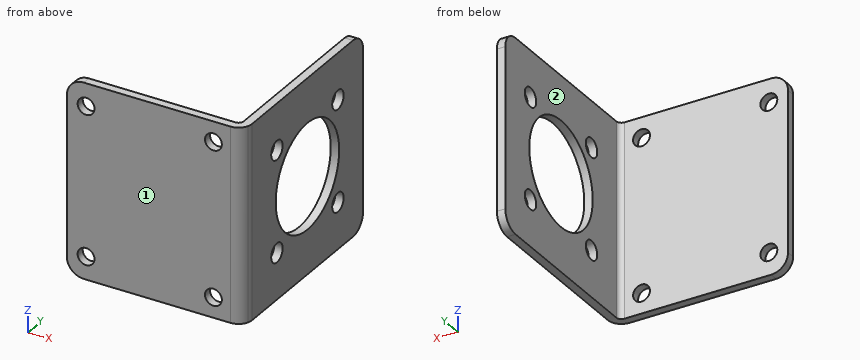
from build123d import *

# Parameters (mm, degrees)
BASE_FLANGE1_DEPTH     = 2
SKETCHED_START         = -23
SKETCHED_BEND1_DEPTH   = 46
SKETCHED_BEND1_2_DEPTH = 46
SKETCH7_R              = 12.5
SKETCH7_R_2            = 2.25
CUT_EXTRUDE1_DEPTH     = 2
SKETCH8_R              = 2
CUT_EXTRUDE2_DEPTH     = 2
FILLET1_R              = 4


# Read off the part's stored shape, not the designer's step: Sketched Bend1
# Sheet-metal steps are written as plain solids
with BuildPart() as part:
    # Sketch1 → Base-Flange1 (new body)
    with BuildSketch(Plane(origin=(0, 0, 0), x_dir=(1, 0, 0), z_dir=(0, 1, 0))):
        Polygon((-20, 23), (20, 23), (66, 23), (66, -23), (20, -23), (-20, -23), align=None)
    extrude(amount=-BASE_FLANGE1_DEPTH)

    # Sketched Bend1 outline → Sketched Bend1 (cut)
    with BuildSketch(Plane.XY.offset(SKETCHED_START)):
        with BuildLine():
            Line((66, 0), (21.766479395, 0))
            ThreePointArc((21.766479395, 0), (20.588854382, -1.453299832), (18.8, -2))
            Line((18.8, -2), (66, -2))
            Line((66, -2), (66, 0))
        make_face()
    extrude(amount=SKETCHED_BEND1_DEPTH, mode=Mode.SUBTRACT)

    # Sketched Bend1 2 outline → Sketched Bend1 2 (add)
    with BuildSketch(Plane.XY.offset(SKETCHED_START)):
        with BuildLine():
            Line((20, 44.944248081), (20, 1.2))
            ThreePointArc((20, 1.2), (19.648528137, 0.351471863), (18.8, 0))
            Line((18.8, 0), (21.766479395, 0))
            ThreePointArc((21.766479395, 0), (21.941077368, 0.58874476), (22, 1.2))
            Line((22, 1.2), (22, 44.944248081))
            Line((22, 44.944248081), (20, 44.944248081))
        make_face()
    extrude(amount=SKETCHED_BEND1_2_DEPTH)

    # Sketch7 → Cut-Extrude1 (cut)
    with BuildSketch(Plane(origin=(22, 0, 0), x_dir=(0, 0, -1), z_dir=(1, 0, 0))):
        with Locations(Location((0, 23, 0), (0, 0, 90))):
            Circle(SKETCH7_R)
        with Locations(Location((12.02081528, 35.02081528, 0), (0, 0, 90))):
            Circle(SKETCH7_R_2)
        with Locations(Location((12.02081528, 10.97918472, 0), (0, 0, 90))):
            Circle(SKETCH7_R_2)
        with Locations(Location((-12.02081528, 10.97918472, 0), (0, 0, 90))):
            Circle(SKETCH7_R_2)
        with Locations(Location((-12.02081528, 35.02081528, 0), (0, 0, 90))):
            Circle(SKETCH7_R_2)
    extrude(amount=-CUT_EXTRUDE1_DEPTH, mode=Mode.SUBTRACT)

    # Sketch8 → Cut-Extrude2 (cut)
    with BuildSketch(Plane(origin=(0, 0, 0), x_dir=(1, 0, 0), z_dir=(0, 1, 0))):
        with Locations(Location((-15.450942979, 17.606788068, 0), (0, 0, 270))):
            Circle(SKETCH8_R)
        with Locations(Location((-15.450942979, -17.606788068, 0), (0, 0, 90))):
            Circle(SKETCH8_R)
        with Locations(Location((14.749785428, 18.198199219, 0), (0, 0, 270))):
            Circle(SKETCH8_R)
        with Locations(Location((14.749785428, -18.198199219, 0), (0, 0, 90))):
            Circle(SKETCH8_R)
    extrude(amount=-CUT_EXTRUDE2_DEPTH, mode=Mode.SUBTRACT)

    # Fillet1
    fillet1_edges = [part.edges().sort_by_distance(p)[0] for p in [
        (21, 44.944248081, -23),
        (21, 44.944248081, 23),
        (-20, -1, 23),
        (-20, -1, -23),
    ]]
    fillet(fillet1_edges, radius=FILLET1_R)


solid = part.part
Model file for the job. Use its own axes, mm. Face numbers are marked on the shaded views. A direction names the side the tool comes from. Give positions to 0.01 mm unless a question says otherwise; leave off trailing zeros. Order: outer loops, then holes, each group sorted by start corner. A loop starts at its lowest first (then second) coordinate and runs counter-clockwise, first axis right, second up. Notation, with made-up numbers: (-1.75, -38.75) - (16.25, -38.75) arc R25 cw to (16.25, -24.75) - close; hole circle Ø9 at (14, -28.75). An arc over 180 degrees is marked (long way). Write item = value, one per line. Start each with the question number.
1. Cut at D-D, the plane y = 31. List the corners of the cut face in (x, z).
2. Which spindle directions (+Z, -Z, +X, -X, +Y, -Y) get a long thin tool onto all of the face, cutting with end or side? Do the marked faces 1 and 2. Say none if no direction does.
3. Cut at A-A, the plane y = 23. List the corners of the cut face in (x, z).
4. Cut at B-B, the plane z = 0. List the corners of the cut face in (x, y), and give its area (3 significant figures).
5. Drop flat-ended pins along their axis: P1, Ø6.5, axis at x = 14.75, z = 18.2, coming from the -Y side; P2, Ø11.5, axis at x = 5, z = 2, coming from the +Y side; P3, Ø5, axis at y = 10.98, z = 12.02, coming from the -X side. Give the stop position or say it passes through.
6. Cut at C-C, the plane x = 18. List the corners of the cut face in (y, z).
7. Probe line 1 along X through (y, z) = (6.5, 5.5); line 2 along Y through (x, z) = (-7.5, -13.5). List the from-to ranges inside material, lowest first.
Taken from the geometry:
q1.outline = (20, -23) - (22, -23) - (22, -9.6) - (20, -9.6) - close; (20, 9.6) - (22, 9.6) - (22, 23) - (20, 23) - close
q2.face_1 = +Z, -Z, +X, -X, -Y
q2.face_2 = +Z, -Z, -X, +Y
q3.outline = (20, -23) - (22, -23) - (22, -12.5) - (20, -12.5) - close; (20, 12.5) - (22, 12.5) - (22, 23) - (20, 23) - close
q4.outline = (-20, -2) - (18.8, -2) arc R3.2 ccw to (22, 1.2) - (22, 10.5) - (20, 10.5) - (20, 1.2) arc R1.2 cw to (18.8, 0) - (-20, 0) - close; (20, 35.5) - (22, 35.5) - (22, 44.94) - (20, 44.94) - close
q4.area = 122 mm²
q5.P1 = -2
q5.P2 = 0
q5.P3 = 20
q6.outline = (-2, -23) - (0, -23) - (0, 23) - (-2, 23) - close
q7.line_1 = 20 to 22
q7.line_2 = -2 to 0
